```python
from build123d import *

# Parameters (mm, degrees)
SKETCH1_R           = 12.5
BOSS_EXTRUDE1_DEPTH = 65
SKETCH3_R           = 2
BOSS_EXTRUDE2_DEPTH = 11
BOSS_EXTRUDE3_DEPTH = 1.5
SKETCH5_W           = 1.5
SKETCH5_H           = 26.3
BOSS_EXTRUDE4_DEPTH = 31
SKETCH6_R           = 4.818685959
SKETCH6_R_2         = 1.6
CUT_EXTRUDE1_DEPTH  = 11


with BuildPart() as part:
    # Sketch1 → Boss-Extrude1 (new body)
    with BuildSketch(Plane(origin=(0, 0, 0), x_dir=(1, 0, 0), z_dir=(0, 1, 0))):
        with Locations(Location((0, 0, 0), (0, 0, 270))):
            Circle(SKETCH1_R)
    extrude(amount=BOSS_EXTRUDE1_DEPTH)

    # Sketch3 → Boss-Extrude2 (add)
    with BuildSketch(Plane(origin=(0, 65, 0), x_dir=(1, 0, 0), z_dir=(0, 1, 0))):
        with Locations(Location((0, 0, 0), (0, 0, 270))):
            Circle(SKETCH3_R)
    extrude(amount=BOSS_EXTRUDE2_DEPTH)

    # Sketch4 → Boss-Extrude3 (add)
    with BuildSketch(Plane(origin=(0, 65, 0), x_dir=(1, 0, 0), z_dir=(0, 1, 0))):
        with BuildLine():
            Line((0, 13.15), (-32, 13.15))
            Line((-32, 13.15), (-32, -13.15))
            Line((-32, -13.15), (0, -13.15))
            ThreePointArc((0, -13.15), (13.15, 0), (0, 13.15))
        make_face()
    extrude(amount=-BOSS_EXTRUDE3_DEPTH)

    # Sketch5 → Boss-Extrude4 (add)
    with BuildSketch(Plane.XZ.offset(-63.5)):
        with Locations((-31.25, 0)):
            Rectangle(SKETCH5_W, SKETCH5_H)
    extrude(amount=BOSS_EXTRUDE4_DEPTH)

    # Sketch6 → Cut-Extrude1 (cut)
    with BuildSketch(Plane.ZY.offset(32)):
        with Locations((0, 49.181314041)):
            Circle(SKETCH6_R)
        with Locations((-8.175, 56.9)):
            Circle(SKETCH6_R_2)
        with Locations((8.175, 56.9)):
            Circle(SKETCH6_R_2)
        with Locations((8.175, 42.6)):
            Circle(SKETCH6_R_2)
        with Locations((-8.175, 42.6)):
            Circle(SKETCH6_R_2)
    extrude(amount=-CUT_EXTRUDE1_DEPTH, mode=Mode.SUBTRACT)


solid = part.part
```
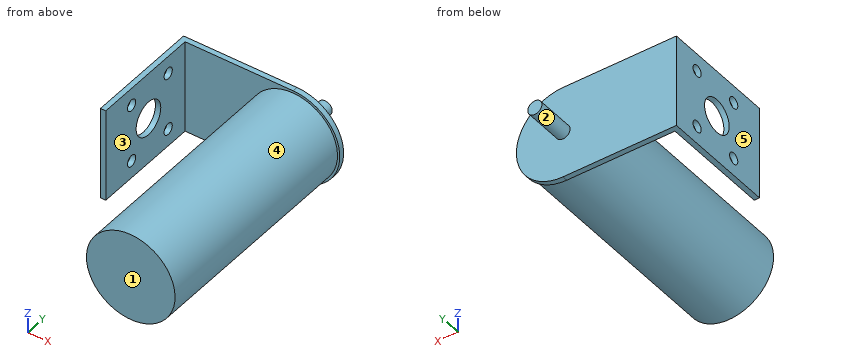
Input: part model. Units: mm. Frame: model coordinates. Face numbers are marked on the shaded views. A direction names the side the tool comes from. Give positions to 0.01 mm unless a question says otherwise; leave off trailing zeros. Order: outer loops, then holes, each group sorted by start corner. A loop starts at its lowest first (then second) coordinate and runs counter-clockwise, first axis right, second up.
1. Section C-C on z = 8.5. Return the cut outline in (x, y), and give its area (3 significant figures).
Derived:
outline: (-32, 32.5) - (-30.5, 32.5) - (-30.5, 41.03) - (-32, 41.03) - close; (-32, 44.17) - (-30.5, 44.17) - (-30.5, 55.33) - (-32, 55.33) - close; (-32, 58.47) - (-30.5, 58.47) - (-30.5, 63.5) - (-9.17, 63.5) - (-9.17, 0) - (9.17, 0) - (9.17, 63.5) - (10.03, 63.5) - (10.03, 65) - (-32, 65) - close
area: 1,260 mm2
2. Section D-D on x = -20. Return the cut outline in (y, z), and give its area (4 significant figures).
Derived:
outline: (63.5, -13.15) - (65, -13.15) - (65, 13.15) - (63.5, 13.15) - close
area: 39.45 mm2
3. Section B-B on y = 56.9. Return the cut outline in (x, z) (3 decimals), and give its area (3 significant figures).
Derived:
outline: (-32, -13.15) - (-30.5, -13.15) - (-30.5, -9.775) - (-32, -9.775) - close; (-32, -6.575) - (-30.5, -6.575) - (-30.5, 6.575) - (-32, 6.575) - close; (-32, 9.775) - (-30.5, 9.775) - (-30.5, 13.15) - (-32, 13.15) - close; circle Ø25 at (0, 0)
area: 521 mm2
4. Mould query, pull axis X, two halves, no side actions, for the marked faces 1, 2 and 3. Classes: released by +X, released by -X, zero draft, split by the parting line, or undercut.
Derived:
face 1: zero draft
face 2: split by the parting line
face 3: undercut
5. Material intervals for L1, parallel to Z at x = -31, y = 42; L2, parallel to Y at x = -14.5, z = -4.75; L3, parallel to Y at x = -31.3, z = 0, sorted ascending.
Derived:
L1: z = -13.15 to -9.66, -6.69 to 6.69, 9.66 to 13.15
L2: y = 63.5 to 65
L3: y = 32.5 to 44.36, 54 to 65
6. Pin query (flat end, axial travel): pin 1 (6 mm diameter, centred on x = 5, y = 37, fed in from -Z); pin 2 (6 mm diameter, centred on x = 1.5, y = 45, fed in from -Z); pin 3 (3 mm diameter, centred on x = -3, z = 7.5, fed in from +Y). Return the tip coordinate at first contact, or that it passes through.
Derived:
pin 1: stops at z = -12.34
pin 2: stops at z = -12.5
pin 3: stops at y = 65
7. Section A-A on z = 0. Return the cut outline in (x, y).
Derived:
outline: (-32, 32.5) - (-30.5, 32.5) - (-30.5, 44.36) - (-32, 44.36) - close; (-32, 54) - (-30.5, 54) - (-30.5, 63.5) - (-12.5, 63.5) - (-12.5, 0) - (12.5, 0) - (12.5, 63.5) - (13.15, 63.5) - (13.15, 65) - (2, 65) - (2, 76) - (-2, 76) - (-2, 65) - (-32, 65) - close
8. Reachability of the marked faces 4 and 5 from +Z, -Z, +X, -X, +Y, -Y: full face, straight path, thin tool, end or side. Return the list, or none.
Derived:
face 4: -Y
face 5: +Z, -Z, -X, +Y, -Y
